```python
from build123d import *

# Parameters (mm, degrees)
F0_R     = 2.575
F1_DEPTH = 2
F2_R     = 3.5
F3_DEPTH = 2
F4_R     = 3.5
F5_DEPTH = 2


with BuildPart() as f1:
    # F0 (on Top) → F1 (new body)
    with BuildSketch(Plane.XY):
        with BuildLine():
            Line((25.175, 25.015), (18.107727, 25.015))
            Line((18.107727, 25.015), (0, 25.015))
            Line((0, 25.015), (-18.107727, 25.015))
            Line((-18.107727, 25.015), (-25.175, 25.015))
            ThreePointArc((-25.175, 25.015), (-27.29632, 24.13632), (-28.175, 22.015))
            Line((-28.175, 22.015), (-28.175, 18.29321))
            Line((-28.175, 18.29321), (-28.175, -18.29321))
            Line((-28.175, -18.29321), (-28.175, -22.015))
            ThreePointArc((-28.175, -22.015), (-27.29632, -24.13632), (-25.175, -25.015))
            Line((-25.175, -25.015), (-18.107727, -25.015))
            Line((-18.107727, -25.015), (0, -25.015))
            Line((0, -25.015), (18.107727, -25.015))
            Line((18.107727, -25.015), (25.175, -25.015))
            ThreePointArc((25.175, -25.015), (27.29632, -24.13632), (28.175, -22.015))
            Line((28.175, -22.015), (28.175, -18.29321))
            Line((28.175, -18.29321), (28.175, 18.29321))
            Line((28.175, 18.29321), (28.175, 22.015))
            ThreePointArc((28.175, 22.015), (27.29632, 24.13632), (25.175, 25.015))
        make_face()
        with Locations((-18.65, -19.44)):
            Circle(F0_R, mode=Mode.SUBTRACT)
        with Locations((18.65, -19.44)):
            Circle(F0_R, mode=Mode.SUBTRACT)
        with Locations((-18.65, 19.44)):
            Circle(F0_R, mode=Mode.SUBTRACT)
        with Locations((18.65, 19.44)):
            Circle(F0_R, mode=Mode.SUBTRACT)
    extrude(amount=F1_DEPTH)

    # F2 (on face) → F3 (join)
    with BuildSketch(Plane(origin=(-28.175, 0, 0), x_dir=(0, -1, 0), z_dir=(-1, 0, 0))):
        with BuildLine():
            Line((-22.015, 2), (19.493148, 2))
            ThreePointArc((19.493148, 2), (-1.260926, 22.754074), (-22.015, 2))
        make_face()
        with Locations((-5.59321, 16)):
            Circle(F2_R, mode=Mode.SUBTRACT)
    extrude(amount=-F3_DEPTH)

    # F4 (on face) → F5 (join)
    with BuildSketch(Plane.YZ.offset(28.175)):
        with BuildLine():
            Line((-19.493, 2), (22.015, 2))
            ThreePointArc((22.015, 2), (1.261, 22.754), (-19.493, 2))
        make_face()
        with Locations((5.593, 16)):
            Circle(F4_R, mode=Mode.SUBTRACT)
    extrude(amount=-F5_DEPTH)


solid = f1.part
```
For this review, take the finished solid that the model builds, in its own axes (mm). A direction names the side the tool comes from. Give positions to 0.01 mm unless a question says otherwise; leave off trailing zeros. Write each loop counter-clockwise with the first axis right and the second up, starting at its lowest first coordinate (ties: lowest second). Pieces come first, ordered by that corner, then holes. Notation, with made-up numbers: M 33.5,84 L 75.5,84 A28 cw 75.5,117 Z; hole C -19.5,-2 d1. An arc over 180 degrees is marked long. Answer as a JSON object with one key per item and string values. Group by question number.
Item 1: Draft analysis for pull direction Y (two halves, no side actions). For faces 3 (the flat face through (0, 0, 2)), 4 (the cylindrical face through (-17.266, -17.269, 0.986)), 5 (the cylindrical face through (27.19, 5.14, 19.47)), 6 (the cylindrical face through (-27.32, -24.11, 0.99)), state which applies: +Y half, -Y half, draft (parallel to the pull), parting line (faces both ways), or undercut.
Item 2: Consider section B-B on z = 9.75. Write out the cut boundary in (x, y) (3 decimals), plus the area to 3 significant figures.
Item 3: For probe 1 along Y at (x, z) = (18.65, 0.9) (3 decimals); probe 2 along X at (y, z) = (1, 21.25) (3 decimals); probe 3 along Z at (x, y) = (-7, -18.5), list the stretches that pass through material, from the lowest coordinate up. Write a range as [from, to].
Item 4: For pin 1 Ø4 at (x, y) = (18.65, 19.44) entering from -Z; pin 2 Ø3 at (x, y) = (-1, -12.5) entering from -Z; pin 3 Ø2 at (x, y) = (-1, 15.5) entering from +Z, all flat-tipped, find the tip position at first contact; note any pin that passes through.
Item 5: Consider section C-C on y = 4. Write out the cut boundary in (x, z) (3 decimals).
Item 6: Tool access review of faces 1 (the flat face through (26.175, 1, 10)), 2 (the cylindrical face through (-27.19, 6.05, 19.47)): name each direction out of +Z, -Z, +X, -X, +Y, -Y from which nothing blocks a thin tool from reaching the whole face with its end or side.
Item 7: Consider section D-D on z = 13.75. Write out the cut boundary in (x, y) (1 decimal).
Item 8: Consider section A-A on x = -18.65. Write out the cut boundary in (y, z) (3 decimals).
Check result:
{
 "1": {"face 3": "draft", "face 4": "undercut", "face 5": "undercut", "face 6": "-Y half"},
 "2": {"outline": "M -28.175,-17.992 L -26.175,-17.992 L -26.175,20.514 L -28.175,20.514 Z; M 26.175,-17.992 L 28.175,-17.992 L 28.175,20.514 L 26.175,20.514 Z", "area": "154 mm^2"},
 "3": {"probe 1": "y = [-25.015, -22.015], [-16.865, 16.865], [22.015, 25.015]", "probe 2": "x = [-28.175, -26.175], [26.175, 28.175]", "probe 3": "z = [0, 2]"},
 "4": {"pin 1": "passes through", "pin 2": "stops at z = 0", "pin 3": "stops at z = 2"},
 "5": {"outline": "M -28.175,0 L 28.175,0 L 28.175,12.884 L 26.175,12.884 L 26.175,2 L -26.175,2 L -26.175,12.884 L -28.175,12.884 Z; M -28.175,19.116 L -26.175,19.116 L -26.175,22.573 L -28.175,22.573 Z; M 26.175,19.116 L 28.175,19.116 L 28.175,22.572 L 26.175,22.572 Z"},
 "6": {"face 1": "+Z, +Y, -Y", "face 2": "+X, -X"},
 "7": {"outline": "M -28.2,-15.8 L -26.2,-15.8 L -26.2,2.9 L -28.2,2.9 Z; M -28.2,8.3 L -26.2,8.3 L -26.2,18.4 L -28.2,18.4 Z; M 26.2,-15.8 L 28.2,-15.8 L 28.2,2.9 L 26.2,2.9 Z; M 26.2,8.3 L 28.2,8.3 L 28.2,18.4 L 26.2,18.4 Z"},
 "8": {"outline": "M -25.015,0 L -22.015,0 L -22.015,2 L -25.015,2 Z; M -16.865,0 L 16.865,0 L 16.865,2 L -16.865,2 Z; M 22.015,0 L 25.015,0 L 25.015,2 L 22.015,2 Z"}
}
